```python
from build123d import *

# Parameters (mm, degrees)
BOSS_EXTRUDE1_DEPTH     = 10
FILLET1_R               = 5
CUT_EXTRUDE1_DEPTH      = 207.767985917
CUT_EXTRUDE1_DEPTH_BACK = 207.767985917
SKETCH2_R               = 3
FILLET2_R               = 1
SKETCH4_R               = 1
CUT_EXTRUDE2_DEPTH      = 207.767985981


with BuildPart() as part:
    # Sketch1 → Boss-Extrude1 (new body)
    with BuildSketch(Plane.XY):
        Polygon((125, 158), (-125, 158), (-133, 158), (-133, 150), (-133, 0), (-133, -8), (-125, -8), (125, -8), (133, -8), (133, 0), (133, 150), (133, 158), align=None)
    extrude(amount=BOSS_EXTRUDE1_DEPTH)

    # Fillet1
    fillet1_edges = [part.edges().sort_by_distance(p)[0] for p in [
        (-133, -8, 5),
        (133, -8, 5),
        (133, 158, 5),
        (-133, 158, 5),
    ]]
    fillet(fillet1_edges, radius=FILLET1_R)

    # Sketch2 → Cut-Extrude1 (cut, two sides: drawn at the far end of the back side and taken through both)
    with BuildSketch(Plane(origin=(0, 0, 0), x_dir=(-1, 0, 0), z_dir=(0, 0, -1)).offset(-CUT_EXTRUDE1_DEPTH_BACK)):
        with Locations(Location((-50, 132.5, 0), (0, 0, 180))):
            Circle(SKETCH2_R)
        with Locations(Location((50, 132.5, 0), (0, 0, 180))):
            Circle(SKETCH2_R)
        with Locations(Location((-50, 17.5, 0), (0, 0, 180))):
            Circle(SKETCH2_R)
        with Locations(Location((50, 17.5, 0), (0, 0, 180))):
            Circle(SKETCH2_R)
    extrude(amount=CUT_EXTRUDE1_DEPTH + CUT_EXTRUDE1_DEPTH_BACK, mode=Mode.SUBTRACT)

    # Fillet2
    fillet2_edges = [part.edges().sort_by_distance(p)[0] for p in [
        (0, -8, 10),
        (0, -8, 0),
        (131.535533906, -6.535533906, 10),
        (-131.535533906, -6.535533906, 10),
        (133, 75, 10),
        (-133, 75, 10),
        (131.535533906, 156.535533906, 10),
        (-131.535533906, 156.535533906, 10),
        (0, 158, 10),
        (131.535533906, -6.535533906, 0),
        (-131.535533906, -6.535533906, 0),
        (-133, 75, 0),
        (133, 75, 0),
        (-131.535533906, 156.535533906, 0),
        (131.535533906, 156.535533906, 0),
        (0, 158, 0),
    ]]
    fillet(fillet2_edges, radius=FILLET2_R)

    # Sketch4 → Cut-Extrude2 (cut, through all)
    with BuildSketch(Plane(origin=(0, 0, 0), x_dir=(-1, 0, 0), z_dir=(0, 0, -1))):
        with Locations((58.5, 132.4)):
            Circle(SKETCH4_R)
        with Locations((-57.5, 132.4)):
            Circle(SKETCH4_R)
    extrude(amount=-CUT_EXTRUDE2_DEPTH, mode=Mode.SUBTRACT)


solid = part.part
```
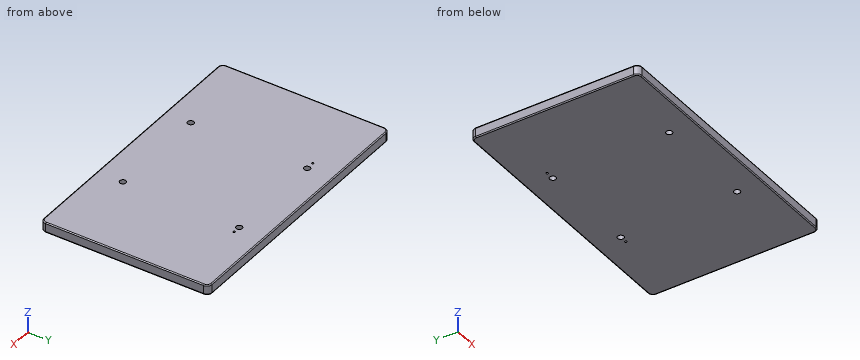
Here's how the part is built. I have some questions about the finished solid (model axes, mm). Round coordinates to 2 decimals unless told otherwise and drop trailing zeros. Write each loop counter-clockwise with the first axis right and the second up, starting at its lowest first coordinate (ties: lowest second). Pieces come first, ordered by that corner, then holes.
Q1. Please list where these lines run through material, in increasing order: probe 1 along X at (y, z) = (132.5, 2); probe 2 along Y at (x, z) = (-50, 2.25); probe 3 along Y at (x, z) = (-58.5, 2.25).
Q2. If we section it at B-B on y = 17.5: Write out the boundary of the cut face in (x, z).
Q3. If we section it at A-A on x = 50: Write out the boundary of the cut face in (y, z).
Answer below:
1. probe 1: x = -133 to -59.49, -57.51 to -53, -47 to 47, 53 to 56.51, 58.49 to 133
1. probe 2: y = -8 to 14.5, 20.5 to 129.5, 135.5 to 158
1. probe 3: y = -8 to 131.4, 133.4 to 158
2. outline: (-133, 1) arc R1 ccw to (-132, 0) - (-53, 0) - (-53, 10) - (-132, 10) arc R1 ccw to (-133, 9) - close; (-47, 0) - (47, 0) - (47, 10) - (-47, 10) - close; (53, 0) - (132, 0) arc R1 ccw to (133, 1) - (133, 9) arc R1 ccw to (132, 10) - (53, 10) - close
3. outline: (-8, 1) arc R1 ccw to (-7, 0) - (14.5, 0) - (14.5, 10) - (-7, 10) arc R1 ccw to (-8, 9) - close; (20.5, 0) - (129.5, 0) - (129.5, 10) - (20.5, 10) - close; (135.5, 0) - (157, 0) arc R1 ccw to (158, 1) - (158, 9) arc R1 ccw to (157, 10) - (135.5, 10) - close
